from build123d import *

# Parameters (mm, degrees)
SKETCH_R        = 17
PAD_DEPTH       = 4
CHAMFER_SIZE    = 1
PAD001_DEPTH    = 10
SKETCH002_R     = 3.5
PAD002_DEPTH    = 3
SKETCH003_R     = 1.5
POCKET_DEPTH    = 6
FILLET_R        = 1
SKETCH004_R     = 3.5
PAD003_DEPTH    = 3
SKETCH005_R     = 1.5
POCKET001_DEPTH = 6
FILLET001_R     = 1


with BuildPart() as part:
    # Sketch → Pad (new body)
    with BuildSketch(Plane.XY):
        with Locations((0, 4.3)):
            Circle(SKETCH_R)
        with BuildLine():
            ThreePointArc((7.8, 8.6), (0, 16.4), (-7.8, 8.6))
            Line((-7.8, 8.6), (-7.8, 0))
            ThreePointArc((-7.8, 0), (0, -7.8), (7.8, 0))
            Line((7.8, 0), (7.8, 8.6))
        make_face(mode=Mode.SUBTRACT)
    extrude(amount=PAD_DEPTH)

    # Chamfer
    chamfer_edges = [part.edges().sort_by_distance(p)[0] for p in [
        (-17, 4.3, 4),
    ]]
    chamfer(chamfer_edges, length=CHAMFER_SIZE)

    # Sketch001 (on Face4 of Chamfer) → Pad001 (join)
    with BuildSketch(Plane.XY.offset(4)):
        with BuildLine():
            ThreePointArc((9.8, 8.6), (0, 18.4), (-9.8, 8.6))
            Line((-9.8, 0), (-9.8, 8.6))
            ThreePointArc((-9.8, 0), (0, -9.8), (9.8, 0))
            Line((9.8, 0), (9.8, 8.6))
        make_face()
        with BuildLine():
            ThreePointArc((7.8, 8.6), (0, 16.4), (-7.8, 8.6))
            Line((-7.8, 0), (-7.8, 8.6))
            ThreePointArc((-7.8, 0), (0.000482, -7.8), (7.8, 0.000965))
            Line((7.8, 0.000965), (7.8, 8.6))
        make_face(mode=Mode.SUBTRACT)
    extrude(amount=PAD001_DEPTH)

    # Sketch002 (on Face10 of Pad001) → Pad002 (join)
    with BuildSketch(Plane(origin=(-9.8, 0, 0), x_dir=(0, -1, 0), z_dir=(-1, 0, 0))):
        with Locations((-4.3, 8)):
            Circle(SKETCH002_R)
    extrude(amount=PAD002_DEPTH)

    # Sketch003 (on Face19 of Pad002) → Pocket (cut)
    with BuildSketch(Plane(origin=(-12.8, 0, 0), x_dir=(0, -1, 0), z_dir=(-1, 0, 0))):
        with Locations((-4.3, 8)):
            Circle(SKETCH003_R)
    extrude(amount=-POCKET_DEPTH, mode=Mode.SUBTRACT)

    # Fillet
    fillet_edges = [part.edges().sort_by_distance(p)[0] for p in [
        (-12.8, 7.8, 8),
    ]]
    fillet(fillet_edges, radius=FILLET_R)

    # Sketch004 (on Face10 of Fillet) → Pad003 (join)
    with BuildSketch(Plane.YZ.offset(9.8)):
        with Locations((4.3, 8)):
            Circle(SKETCH004_R)
    extrude(amount=PAD003_DEPTH)

    # Sketch005 (on Face22 of Pad003) → Pocket001 (cut)
    with BuildSketch(Plane.YZ.offset(12.8)):
        with Locations((4.3, 8)):
            Circle(SKETCH005_R)
    extrude(amount=-POCKET001_DEPTH, mode=Mode.SUBTRACT)

    # Fillet001
    fillet001_edges = [part.edges().sort_by_distance(p)[0] for p in [
        (12.8, 0.8, 8),
    ]]
    fillet(fillet001_edges, radius=FILLET001_R)


solid = part.part
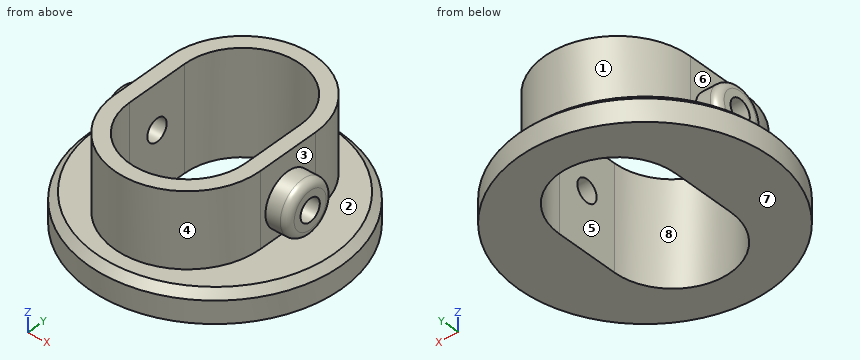
Here's how the part is built. I have some questions about the finished solid (model axes, mm). Face numbers are marked on the shaded views. A direction names the side the tool comes from. Give positions to 0.01 mm unless a question says otherwise; leave off trailing zeros. Loops run counter-clockwise (first coordinate to the right, second up) from the corner with the lowest first, then second, coordinate; pieces in that order, holes last. Notation, with made-up numbers: (-31, 54.25) -> (19, 54.25) arc R26 cw to (19, 82.25) -> close; hole circle Ø6 at (-27.5, 13). An arc over 180 degrees is marked (long way). Answer as a JSON object with one key per item and string values. Group by question number.
Item 1: Imagine slicing it at A-A on y = 4.3. Give the number of separate pieces and of enclosed holes in the cut face, then the cut area to 3 significant figures.
Item 2: I need wall thicknesses on L1, parallel to Z at x = -11, y = 4.3; L2, parallel to X at y = 6.5, z = 13; L3, parallel to Z at x = -9.7, y = 4.3. Which ranges of each line are inside material? Lowest first, please.
Item 3: On a 3-axis mill with a long thin cutter (end or side, diameter ignored), from which of +Z, -Z, +X, -X, +Y, -Y can I reach the whole of each face in a straight line? I mean the marked faces 1, 2, 3, 4 and 5. Say none if no direction works.
Item 4: Imagine slicing it at B-B on z = 8. Write out the boundary of the cut face in (x, y), then the cut area to 3 significant figures.
Item 5: Thinking about a two-plate mould opening in Z: for the marked faces 6, 7 and 8, which applies, pulls with the +Z half, pulls with the -Z half, needs draft (parallel to the pull), parting line crosses it, or undercut?
Item 6: Will these pins go through, and if not, where does the flat tip stop? pin 1 (4 mm diameter, centred on y = 5.5, z = 9, fed in from -X); pin 2 (4 mm diameter, centred on y = 4, z = 7, fed in from +X); pin 3 (1 mm diameter, centred on y = 14.5, z = 10, fed in from -X).
Answer list:
{
 "1": {"separate pieces": "4", "enclosed holes": "0", "area": "124 mm2"},
 "2": {"L1": "z = 0 to 4, 4.5 to 6.5, 9.5 to 11.5", "L2": "x = -9.8 to -7.8, 7.8 to 9.8", "L3": "z = 0 to 6.5, 9.5 to 14"},
 "3": {"face 1": "+Z, +Y", "face 2": "none", "face 3": "+X", "face 4": "+Z, -Y", "face 5": "+Z, -Z"},
 "4": {"outline": "(-12.8, 1.8) arc R1 ccw to (-11.8, 0.8) -> (-9.8, 0.8) -> (-9.8, 0) arc R9.8 ccw to (9.8, 0) -> (9.8, 0.8) -> (11.8, 0.8) arc R1 ccw to (12.8, 1.8) -> (12.8, 2.8) -> (7.8, 2.8) -> (7.8, 0) arc R7.8 cw to (-7.8, 0) -> (-7.8, 2.8) -> (-12.8, 2.8) -> close; (-12.8, 5.8) -> (-7.8, 5.8) -> (-7.8, 8.6) arc R7.8 cw to (7.8, 8.6) -> (7.8, 5.8) -> (12.8, 5.8) -> (12.8, 6.8) arc R1 ccw to (11.8, 7.8) -> (9.8, 7.8) -> (9.8, 8.6) arc R9.8 ccw to (-9.8, 8.6) -> (-9.8, 7.8) -> (-11.8, 7.8) arc R1 ccw to (-12.8, 6.8) -> close", "area": "156 mm2"},
 "5": {"face 6": "undercut", "face 7": "pulls with the -Z half", "face 8": "needs draft"},
 "6": {"pin 1": "stops at x = -12.8", "pin 2": "stops at x = 12.8", "pin 3": "stops at x = -8.18"}
}
